Read the model definition and answer for the solid it produces. Units are mm, in the model's axes. Coordinates: 2 decimals unless noted, no trailing zeros. Loops run counter-clockwise (first coordinate to the right, second up) from the corner with the lowest first, then second, coordinate; pieces in that order, holes last. Notation, with made-up numbers: M 9.5,1 L 63.5,1 A10 ccw 63.5,10 Z; hole C 3.25,-14 d5. An arc over 180 degrees is marked long. Use one line per item in the form item = value. Start each with the question number.
1. Find the intervals of material crossed by probe 1 along X at (y, z) = (-10.5, -16.5); probe 2 along X at (y, z) = (-44, -19); probe 3 along Z at (x, y) = (37, -22.5), in increasing order. Write a range as [from, to].
2. The part is cut by section A-A (y = -23.5). Give the vertices of the cut face in (x, z) (3 decimals).
3. Flat-ended cylindrical pins translate along their axes: pin 1 (2 mm diameter, centred on y = -10, z = 7, fed in from -X); pin 2 (8.5 mm diameter, centred on x = -53.5, y = -20, fed in from -Z); pin 3 (5.5 mm diameter, centred on x = 35.79, z = -20.15, fed in from -Y). Find the tip coordinate at first contact, or state that the pin passes through.
4. The part is cut by section B-B (z = 11). Give the vertices of the cut face in (x, y), plus the area to 3 significant figures.
5. For a pull along X with two mould halves and no side action, classify faces 1 (the flat face through (-53, -25, -20.754)), 2 (the flat face through (-50.17, -25.044, 12.124)), 3 (the cylindrical face through (34.83, -25.044, -24.492)) as released by +X, released by -X, zero draft, split by the parting line, or undercut.
from build123d import *

# Parameters (mm, degrees)
F0_R     = 4.445
F1_DEPTH = 50.8


with BuildPart() as f1:
    # F0 (on Front) → F1 (new body)
    with BuildSketch(Plane.XZ):
        Polygon((53.841315, 18.648949), (-35.19237, 18.648949), (-65.572105, 5.414211), (-65.572105, -13.836316), (-61.060261, -20.754473), (-43.915264, -20.754473), (-35.19237, -25.567105), (53.841315, -25.567105), (71.888685, -18.047368), (76.701313, -8.722895), (71.888685, 5.414211), align=None)
        with Locations((-20.754473, -20.152895)):
            Circle(F0_R, mode=Mode.SUBTRACT)
        with Locations((35.793949, -20.152895)):
            Circle(F0_R, mode=Mode.SUBTRACT)
    extrude(amount=F1_DEPTH)


solid = f1.part
Computed values:
q1.probe_1 = [-63.83, -23.29], [-18.22, 33.26], [38.33, 72.69]
q1.probe_2 = [-62.2, -25.05], [-16.46, 31.5], [40.09, 69.6]
q1.probe_3 = [-25.57, -24.43], [-15.87, 18.65]
q2.outline = M -65.572,-13.836 L -61.06,-20.754 L -43.915,-20.754 L -35.192,-25.567 L 53.841,-25.567 L 71.889,-18.047 L 76.701,-8.723 L 71.889,5.414 L 53.841,18.649 L -35.192,18.649 L -65.572,5.414 Z; hole C -20.754,-20.153 d8.89; hole C 35.794,-20.153 d8.89
q3.pin_1 = -64.23
q3.pin_2 = -20.75
q3.pin_3 = through
q4.outline = M -52.75,-50.8 L 64.27,-50.8 L 64.27,0 L -52.75,0 Z
q4.area = 5,940 mm²
q5.face_1 = zero draft
q5.face_2 = released by -X
q5.face_3 = undercut
